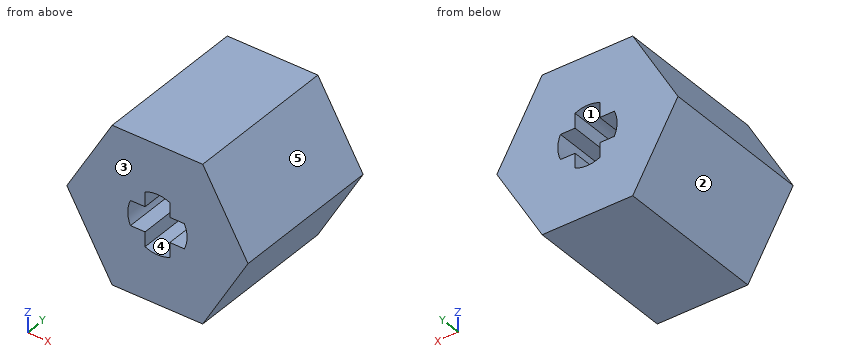
```python
from build123d import *

# Parameters (mm, degrees)
SKETCH1_R           = 2.4
BOSS_EXTRUDE1_DEPTH = 12.5


with BuildPart() as part:
    # Sketch1 → Boss-Extrude1 (new body)
    # profile 1 of 5: a face of its own
    with BuildSketch(Plane(origin=(0, 0, 0), x_dir=(1, 0, 0), z_dir=(0, 1, 0))):
        Polygon((-3.666174209, -6.35), (3.666174209, -6.35), (7.332348419, 0), (3.666174209, 6.35), (-3.666174209, 6.35), (-7.332348419, 0), align=None)
        Circle(SKETCH1_R, mode=Mode.SUBTRACT)
    # profile 2 of 5: a face of its own
    with BuildSketch(Plane(origin=(0, 0, 0), x_dir=(1, 0, 0), z_dir=(0, 1, 0))):
        with BuildLine():
            Line((-2.181742423, 1), (-1, 1))
            Line((-1, 1), (-1, 2.181742423))
            ThreePointArc((-1, 2.181742423), (-1.697056275, 1.697056275), (-2.181742423, 1))
        make_face()
    # profile 3 of 5: a face of its own
    with BuildSketch(Plane(origin=(0, 0, 0), x_dir=(1, 0, 0), z_dir=(0, 1, 0))):
        with BuildLine():
            Line((-1, -2.181742423), (-1, -1))
            Line((-1, -1), (-2.181742423, -1))
            ThreePointArc((-2.181742423, -1), (-1.697056275, -1.697056275), (-1, -2.181742423))
        make_face()
    # profile 4 of 5: a face of its own
    with BuildSketch(Plane(origin=(0, 0, 0), x_dir=(1, 0, 0), z_dir=(0, 1, 0))):
        with BuildLine():
            Line((2.181742423, -1), (1, -1))
            Line((1, -1), (1, -2.181742423))
            ThreePointArc((1, -2.181742423), (1.697056275, -1.697056275), (2.181742423, -1))
        make_face()
    # profile 5 of 5: a face of its own
    with BuildSketch(Plane(origin=(0, 0, 0), x_dir=(1, 0, 0), z_dir=(0, 1, 0))):
        with BuildLine():
            Line((1, 2.181742423), (1, 1))
            Line((1, 1), (2.181742423, 1))
            ThreePointArc((2.181742423, 1), (1.697056275, 1.697056275), (1, 2.181742423))
        make_face()
    extrude(amount=BOSS_EXTRUDE1_DEPTH)


solid = part.part
```
Source: CAD feature listing. Evaluate the final solid. Frame: model axes, mm. Face numbers are marked on the shaded views. A direction names the side the tool comes from. Coordinates: 2 decimals unless noted, no trailing zeros. Loops run counter-clockwise (first coordinate to the right, second up) from the corner with the lowest first, then second, coordinate; pieces in that order, holes last. Notation, with made-up numbers: (39, 55) -> (69, 55) arc R17 cw to (69, 88) -> close; hole circle Ø6 at (67, 9.25). An arc over 180 degrees is marked (long way). One line per item, written item: value. Start each with the question number.
Q1. Section query C-C, the plane z = -1.5. Return the cut outline in (x, y), and give its area (3 significant figures).
Q2. Line query: line 1 along Z through (x, y) = (-2, 11); line 2 along X through (y, z) = (6.75, 1.75); line 3 along Z through (x, y) = (-0.75, 7). Output: solid intervals per line, ascending.
Q3. Section query D-D, the plane x = 5.75. Return the cut outline in (y, z), and give its area (3 significant figures).
Q4. Contact query for flat-ended pins moving along their axis: P1, Ø3, axis at x = 2.5, z = 2, coming from the -Y side; P2, Ø0.6, axis at y = 6.5, z = 1.5, coming from the +X side; P3, Ø1.3, axis at y = 8, z = 1.5, coming from the -X side; P4, Ø1, axis at y = 9, z = 1, coming from the +X side. Output: stop coordinate, or through.
Q5. Section query A-A, the plane x = -1.5. Return the cut outline in (y, z), and give its area (3 significant figures).
Q6. Set-up query: the marked faces 4 and 5. Return all of +Z, -Z, +X, -X, +Y, -Y with unobstructed straight access to the full face (end or side cutting, diameter ignored); none if empty.
Q7. Section query B-B, the plane y = 10. Return the cut outline in (x, z), and give its area (3 significant figures).
Q8. Mould query, pull axis X, two halves, no side actions, for the marked faces 1, 2 and 3. Classes: pulls with the +X half, pulls with the -X half, needs draft (parallel to the pull), parting line crosses it, or undercut.
Results:
1. outline: (-6.47, 0) -> (-1, 0) -> (-1, 12.5) -> (-6.47, 12.5) -> close; (1, 0) -> (6.47, 0) -> (6.47, 12.5) -> (1, 12.5) -> close
1. area: 137 mm^2
2. line 1: -6.35 to -1, 1 to 6.35
2. line 2: -6.32 to -1, 1 to 6.32
2. line 3: -6.35 to -2.28, 2.28 to 6.35
3. outline: (0, -2.74) -> (12.5, -2.74) -> (12.5, 2.74) -> (0, 2.74) -> close
3. area: 68.5 mm^2
4. P1: y = 0
4. P2: x = 6.64
4. P3: x = -6.84
4. P4: x = 7.04
5. outline: (0, -6.35) -> (12.5, -6.35) -> (12.5, -1) -> (0, -1) -> close; (0, 1) -> (12.5, 1) -> (12.5, 6.35) -> (0, 6.35) -> close
5. area: 134 mm^2
6. face 4: +Y, -Y
6. face 5: +Z, +X, +Y, -Y
7. outline: (-7.33, 0) -> (-3.67, -6.35) -> (3.67, -6.35) -> (7.33, 0) -> (3.67, 6.35) -> (-3.67, 6.35) -> close; hole (-2.18, -1) -> (-1, -1) -> (-1, -2.18) arc R2.4 ccw to (1, -2.18) -> (1, -1) -> (2.18, -1) arc R2.4 ccw to (2.18, 1) -> (1, 1) -> (1, 2.18) arc R2.4 ccw to (-1, 2.18) -> (-1, 1) -> (-2.18, 1) arc R2.4 ccw to start
7. area: 125 mm^2
8. face 1: undercut
8. face 2: pulls with the -X half
8. face 3: needs draft
